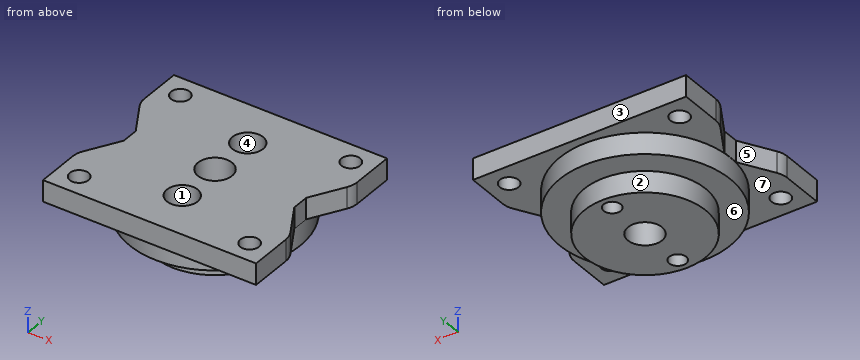
Autodesk Inventor part; units mm, degrees
ref_plane "Work Plane1" through (0, 0, 0) normal (0, 0, 1) x (1, 0, 0)
ref_plane "Work Plane2" through (-27.0849, -13.97, -71.335) normal (0, 1, 0) x (0, 0, 1)
ref_plane "YZ Plane" through (0, 0, 0) normal (1, 0, 0) x (0, 1, 0)
ref_plane "Work Plane1" through (0, 0, 0) normal (0, 0, 1) x (1, 0, 0)
sketch "Sketch1" plane through (0, 0, 0) normal (0, 0, 1) x (1, 0, 0)
  circle A0 centre (0, 0) radius 9.525
  circle A1 centre (0, 0) radius 12.7
  point P0 (0, 0)
extrude "Extrusion1" add sketch "Sketch1" along normal blind 3.175 contours A0 | A1
sketch "Sketch2" plane through (0, 0, 0) normal (0, 0, -1) x (-1, 0, 0)
  circle A0 centre (0, 0) radius 9.025
  point P0 (0, 0)
  dimension "d2" = 18.05
extrude "Extrusion2" add sketch "Sketch2" along normal blind 3.175
sketch "Sketch3" plane through (0, 0, 3.175) normal (0, 0, 1) x (1, 0, 0)
  circle A0 centre (0, 0) radius 2.54
  point P0 (0, 0)
  dimension "d5" = 5.08
extrude "Extrusion3" cut sketch "Sketch3" against normal through all
sketch "Sketch4" plane through (0, 0, 0) normal (0, 1, 0) x (-1, 0, 0)
  line L0 (12.7, 3.175) -> (-12.7, 3.175)
  line L1 (-12.7, 3.175) -> (12.7, 3.175)
  line L2 (12.7, 3.175) -> (12.7, 6.35)
  line L3 (12.7, 6.35) -> (-12.7, 6.35)
  line L4 (-12.7, 6.35) -> (-12.7, 3.175)
  point P0 (0, 0)
  dimension "d8" = 3.175
ref_plane "Work Plane2" through (-27.0849, -13.97, -71.335) normal (0, 1, 0) x (0, 0, 1)
extrude "Extrusion4" add sketch "Sketch4" against normal up to surface (13.97 mm away)
sketch "Sketch5" plane through (0, 0, 3.175) normal (0, 0, 1) x (1, 0, 0)
  line L0 (-12.7, 0) -> (-2.54, 0)
  arc A0 (2.54, 0) -> (-2.54, 0) centre (0, 0) ccw
  line L1 (2.54, 0) -> (12.7, 0)
  arc A1 (12.7, 0) -> (-12.7, 0) centre (0, 0) ccw
  point P0 (0, 0)
extrude "Extrusion5" add sketch "Sketch5" along normal blind 3.175
sketch "Sketch6" plane through (0, 0, 6.35) normal (0, 0, 1) x (1, 0, 0)
  circle A0 centre (0, 0) radius 1.905
  point P0 (0, 0)
extrude "Extrusion6" cut sketch "Sketch6" against normal blind 3.175
sketch "Sketch8" plane through (0, 0, 3.175) normal (0, 0, -1) x (-1, 0, 0)
  line L0 (-29.0812, -13.97) -> (27.0849, -13.97)
  arc A0 (-1.905, 0) -> (1.905, 0) centre (0, 0) ccw
  arc A1 (12.7, 0) -> (-12.7, 0) centre (0, 0) ccw
  line L1 (12.7, 0) -> (12.7, -13.97)
  line L2 (-12.7, -13.97) -> (12.7, -13.97)
  line L3 (-12.7, 0) -> (-12.7, -13.97)
  line L4 (15.875, -13.97) -> (15.875, -7.62)
  line L5 (15.4496, -6.0325) -> (12.7, -1.27)
  line L6 (12.7, 0) -> (12.7, -13.97)
  arc A2 (15.875, -7.62) -> (15.4496, -6.0325) centre (12.7, -7.62) ccw
  line L7 (-15.875, -13.97) -> (-15.875, -7.62)
  line L8 (-15.4496, -6.0325) -> (-12.7, -1.27)
  line L9 (-12.7, 0) -> (-12.7, -13.97)
  arc A3 (-15.4496, -6.0325) -> (-15.875, -7.62) centre (-12.7, -7.62) ccw
  line L10 (2.54, 0) -> (1.905, 0)
  arc A4 (2.54, 0) -> (-2.54, 0) centre (0, 0) ccw
  line L11 (-1.905, 0) -> (-2.54, 0)
  point P0 (0, 0)
  dimension "d21" = 3.175
  dimension "d22" = 3.175
  dimension "d23" = 6.35
  dimension "d24" = 3.175
  dimension "d25" = 3.175
  dimension "d26" = 6.35
extrude "Extrusion8" add sketch "Sketch8" against normal blind 3.175 contours L7 A3 L8 L3 L0 | L1 L5 A2 L4 L0
sketch "Sketch9" plane through (0, 0, 3.175) normal (0, 0, -1) x (-1, 0, 0)
  circle A0 centre (12.7, -10.795) radius 1.397
  circle A1 centre (-12.7, -10.795) radius 1.397
  line L0 (15.875, -13.97) -> (15.875, -7.62)
  line L1 (-15.875, -13.97) -> (15.875, -13.97)
  line L2 (-15.875, -7.62) -> (-15.875, -13.97)
  point P0 (0, 0)
  dimension "d29" = 3.175
  dimension "d30" = 3.175
  dimension "d31" = 2.794
  dimension "d32" = 3.175
  dimension "d33" = 3.175
extrude "Extrusion9" cut sketch "Sketch9" against normal blind 3.175
sketch "Sketch10" plane through (0, 0, 6.35) normal (0, 0, 1) x (1, 0, 0)
  circle A0 centre (0, 0) radius 2.54
  circle A1 centre (0, 6.985) radius 2.286
  circle A2 centre (0, -6.985) radius 2.286
  circle A3 centre (0, 0) radius 9.025
  dimension "d36" = 5.08
  dimension "d37" = 4.572
  dimension "d38" = 4.572
  dimension "d39" = 6.985
  dimension "d40" = 6.985
extrude "Extrusion10" cut sketch "Sketch10" against normal through all contours A0
extrude "Extrusion11" cut sketch "Sketch10" against normal blind 5.5563 contours A1 A3 | A3 A1 | A3 A2 | A2 A3
sketch "Sketch11" plane through (0, 0, -3.175) normal (0, 0, -1) x (-1, 0, 0)
  circle A0 centre (0, -6.985) radius 2.286
  circle A1 centre (0, 6.985) radius 2.286
  circle A2 centre (0, -6.985) radius 1.27
  circle A3 centre (0, 6.985) radius 1.27
  point P0 (0, 0)
  dimension "d45" = 2.54
extrude "Extrusion12" cut sketch "Sketch11" against normal through all contours A2 | A3
mirror "Mirror1" about plane through (0, 0, 0) normal (0, 1, 0) of "Extrusion8", "Extrusion9", "Extrusion4", "Extrusion11", "Extrusion3", "Extrusion10"
sketch "Sketch12" plane through (-15.875, -13.97, 6.35) normal (0, 0, 1) x (1, 0, 0)
  circle A0 centre (15.875, 13.97) radius 2.2303
extrude "Extrusion13" cut sketch "Sketch12" against normal blind 25.4
properties part number "Cap Top Cap"
The model under review builds one solid part; all positions refer to its coordinate system, in mm. Face numbers are marked on the shaded views. A direction names the side the tool comes from. Give positions to 0.01 mm unless a question says otherwise; leave off trailing zeros. Loops run counter-clockwise (first coordinate to the right, second up) from the corner with the lowest first, then second, coordinate; pieces in that order, holes last. Notation, with made-up numbers: (-21, 85) -> (27, 85) arc R4 ccw to (27, 91) -> close; hole circle Ø8 at (-34.75, 57.5). An arc over 180 degrees is marked (long way). Answer as a JSON object with one key per item and string values. Group by question number.
Q1. Take a section at B-B (y = -0.5). Write out the cut boundary in (x, z) (3 decimals).
Q2. Draft analysis for pull direction X (two halves, no side actions). For the marked faces 1, 2 and 3, state which applies: pulls with the +X half, pulls with the -X half, needs draft (parallel to the pull), parting line crosses it, or undercut.
Q3. Tool access review of the marked faces 4, 5, 6 and 7: name each direction out of +Z, -Z, +X, -X, +Y, -Y from which nothing blocks a thin tool from reaching the whole face with its end or side.
Q4. Take a section at C-C (z = 5.75). Write out the cut boundary in (x, y) (1 decimal), plus the area to 3 significant figures.
Q5. Take a section at D-D (x = -9.5). Write out the cut boundary in (y, z) (3 decimals).
Q6. Wall thickness on line 1 along Y through (x, z) = (0, 4.2); line 2 along Y through (x, z) = (0, -0.95) (3 decimals); line 3 along X through (y, z) = (-11, 5.25) (3 decimals): over which ranges is each line inside the solid? List them lowest first.
Q7. Insertion check: pin 1 (1.4 mm diameter, centred on x = 1, y = -6, fed in from +Z); pin 2 (4 mm diameter, centred on x = -10, z = 1, fed in from +Y); pin 3 (2 mm diameter, centred on y = 0, z = 4, fed in from -X). Each pin has a flat end and moves straight along its axis. Give the tip position at first contact, or say it passes through.
Q8. Take a section at A-A (x = 0). State how many separate pieces and enclosed holes the cut face has, plus the area to 3 significant figures.
Answer below:
{
 "1": {"outline": "(-12.7, 3.175) -> (-12.69, 3.175) -> (-12.69, 0) -> (-9.011, 0) -> (-9.011, -3.175) -> (-2.49, -3.175) -> (-2.49, 6.35) -> (-12.7, 6.35) -> close; (2.49, -3.175) -> (9.011, -3.175) -> (9.011, 0) -> (12.69, 0) -> (12.69, 3.175) -> (12.7, 3.175) -> (12.7, 6.35) -> (2.49, 6.35) -> close"},
 "2": {"face 1": "undercut", "face 2": "parting line crosses it", "face 3": "needs draft"},
 "3": {"face 4": "+Z", "face 5": "+Z, -Z, -X", "face 6": "-Z", "face 7": "-Z, -Y"},
 "4": {"outline": "(-15.9, -14) -> (15.9, -14) -> (15.9, -7.6) arc R3.2 ccw to (15.4, -6) -> (12.7, -1.3) -> (12.7, 1.3) -> (15.4, 6) arc R3.2 ccw to (15.9, 7.6) -> (15.9, 14) -> (-15.9, 14) -> (-15.9, 7.6) arc R3.2 ccw to (-15.4, 6) -> (-12.7, 1.3) -> (-12.7, -1.3) -> (-15.4, -6) arc R3.2 ccw to (-15.9, -7.6) -> close; hole circle Ø2.8 at (-12.7, -10.8); hole circle Ø2.8 at (-12.7, 10.8); hole circle Ø5.1 at (0, 0); hole circle Ø4.6 at (0, -7); hole circle Ø4.6 at (0, 7); hole circle Ø2.8 at (12.7, -10.8); hole circle Ø2.8 at (12.7, 10.8)", "area": "758 mm2"},
 "5": {"outline": "(-13.97, 3.175) -> (-8.429, 3.175) -> (-8.429, 0) -> (8.429, 0) -> (8.429, 3.175) -> (13.97, 3.175) -> (13.97, 6.35) -> (-13.97, 6.35) -> close"},
 "6": {"line 1": "y = -13.97 to -9.27, -4.7 to -2.54, 2.54 to 4.7, 9.27 to 13.97", "line 2": "y = -9.025 to -8.255, -5.715 to -2.54, 2.54 to 5.715, 8.255 to 9.025", "line 3": "x = -15.875 to -14.082, -11.318 to 11.318, 14.082 to 15.875"},
 "7": {"pin 1": "stops at z = 0.79", "pin 2": "stops at y = 9.86", "pin 3": "stops at x = -12.7"},
 "8": {"separate pieces": "4", "enclosed holes": "0", "area": "107 mm2"}
}
